Input: part model. Units: mm. Frame: model coordinates. A direction names the side the tool comes from. Coordinates: 2 decimals unless noted, no trailing zeros. Write each loop counter-clockwise with the first axis right and the second up, starting at its lowest first coordinate (ties: lowest second). Pieces come first, ordered by that corner, then holes. Notation, with made-up numbers: (48, 0) - (56, 0) arc R34 ccw to (56, 36) - close; hole circle Ø9 at (20.25, 25.25). An arc over 180 degrees is marked (long way). Use a Markdown table: item, result. Add a question column.
Q1. Pin query (flat end, axial travel): P1, Ø1.5, axis at y = 1.5, z = -10, coming from the +X side; P2, Ø0.7, axis at y = 8, z = 34.5, coming from the +X side; P3, Ø1.6, axis at x = 51, y = 0.5, coming from the -Z side. Return the tip coordinate at first contact, or that it passes through.
Q2. Section query B-B (x = 12). Return the cut outline in (y, z).
Q3. Mould query, pull axis Z, two halves, no side actions, for faces 4 (the face through (-14, 17.76, 34)), 5 (the face through (60.116, 10.483, 34.289)), 6 (the face through (-36, 1, -11)), 7 (the face through (35, 3.36, 23)). Classes: released by +Z, released by -Z, zero draft, split by the parting line, or undercut.
Q4. Set-up query: faces 1 (the face through (-39, 1, -5.32)), 2 (the face through (-52, 5.76, 23)), 3 (the face through (-57.11, 1.66, -19.82)). Return all of +Z, -Z, +X, -X, +Y, -Y with unobstructed straight access to the full face (end or side cutting, diameter ignored); none if empty.
Q5. Section query A-A (z = 6). Return the cut outline in (x, y).
Q6. Material intervals for probe 1 along Z at (x, y) = (-6.5, 11.75); probe 2 along Z at (x, y) = (30, 6.5); probe 3 along X at (y, z) = (16.75, 16), sorted ascending. Write a range as from..to.
Q7. Section query C-C (x = -40). Return the cut outline in (y, z).
Q8. Section query D-D (x = -24). Return the cut outline in (y, z).
from build123d import *

# Parameters (mm, degrees)
SKETCH_1_W           = 123.84
SKETCH_1_H           = 72
EXTRUDE_1_DEPTH      = 17.76
SKETCH_8_W           = 119.04
SKETCH_8_H           = 67.2
CUT_EXTRUDE_5_DEPTH  = 15.36
SKETCH_10_W          = 54.72
SKETCH_10_H          = 33.6
EXTRUDE_2_DEPTH      = 9.64
SKETCH_11_W          = 15
SKETCH_11_H          = 10.56
CUT_EXTRUDE_7_DEPTH  = 5
SKETCH_12_W          = 51.36
SKETCH_12_H          = 30.24
CUT_EXTRUDE_8_DEPTH  = 7
SKETCH_13_W          = 24.6
SKETCH_13_H          = 20.96
CUT_EXTRUDE_9_DEPTH  = 2
CUT_EXTRUDE_16_DEPTH = 73.428336996
FILLET_1_R           = 6
FILLET_3_R           = 3
FILLET_5_R           = 6
SKETCH_19_W          = 5.5
SKETCH_19_H          = 2
CUT_EXTRUDE_14_DEPTH = 3.84
SKETCH_20_W          = 5.5
SKETCH_20_H          = 2
CUT_EXTRUDE_15_DEPTH = 3.84
EXTRUDE_3_DEPTH      = 3.36
EXTRUDE_4_DEPTH      = 3.36
SKETCH_25_R          = 2.16
SKETCH_25_R_2        = 2.26
CUT_EXTRUDE_17_DEPTH = 74.793658264
SKETCH_22_R          = 3.71
SKETCH_22_R_2        = 3.12
CUT_EXTRUDE_18_DEPTH = 3.36
SKETCH_26_W          = 24.96
SKETCH_26_H          = 11.04
SKETCH_26_W_2        = 3.84
SKETCH_26_H_2        = 1.92
SKETCH_26_W_3        = 8.16
SKETCH_26_H_3        = 8.16
CUT_EXTRUDE_19_DEPTH = 74.793658264


with BuildPart() as part:
    # Эскиз1 → Бобышка-Вытянуть1 (new body)
    with BuildSketch(Plane(origin=(0, 0, 0), x_dir=(1, 0, 0), z_dir=(0, 1, 0))):
        Rectangle(SKETCH_1_W, SKETCH_1_H)
    extrude(amount=EXTRUDE_1_DEPTH)

    # Эскиз8 → Вырез-Вытянуть5 (cut)
    with BuildSketch(Plane(origin=(0, 17.76, 0), x_dir=(1, 0, 0), z_dir=(0, 1, 0))):
        Rectangle(SKETCH_8_W, SKETCH_8_H)
    extrude(amount=-CUT_EXTRUDE_5_DEPTH, mode=Mode.SUBTRACT)

    # Эскиз10 → Бобышка-Вытянуть2 (add)
    with BuildSketch(Plane(origin=(0, 2.4, 0), x_dir=(1, 0, 0), z_dir=(0, 1, 0))):
        with Locations((14.88, -2.2)):
            Rectangle(SKETCH_10_W, SKETCH_10_H)
    extrude(amount=EXTRUDE_2_DEPTH)

    # Эскиз11 → Вырез-Вытянуть7 (cut)
    with BuildSketch(Plane.XY.offset(33.6)):
        with Locations((-42.42, 9.12)):
            Rectangle(SKETCH_11_W, SKETCH_11_H)
    extrude(amount=CUT_EXTRUDE_7_DEPTH, mode=Mode.SUBTRACT)

    # Эскиз12 → Вырез-Вытянуть8 (cut)
    with BuildSketch(Plane.XZ):
        with Locations((14.64, 2.44)):
            Rectangle(SKETCH_12_W, SKETCH_12_H)
    extrude(amount=-CUT_EXTRUDE_8_DEPTH, mode=Mode.SUBTRACT)

    # Эскиз13 → Вырез-Вытянуть9 (cut)
    with BuildSketch(Plane.XZ):
        with Locations((49.62, 2.28)):
            Rectangle(SKETCH_13_W, SKETCH_13_H)
    extrude(amount=-CUT_EXTRUDE_9_DEPTH, mode=Mode.SUBTRACT)

    # Эскиз21 → Вырез-Вытянуть16 (cut, through all)
    with BuildSketch(Plane.XZ.offset(-7)):
        Polygon((-1.44, 7.24), (-1.44, -2.04), (-11.04, -2.04), (-11.04, 2.44), (-11.04, 7.24), align=None)
    extrude(amount=-CUT_EXTRUDE_16_DEPTH, mode=Mode.SUBTRACT)

    # Скругление1
    fillet_1_edges = [part.edges().sort_by_distance(p)[0] for p in [
        (-61.92, 8.88, -36),
        (61.92, 8.88, -36),
        (61.92, 8.88, 36),
        (-61.92, 8.88, 36),
    ]]
    fillet(fillet_1_edges, radius=FILLET_1_R)

    # Скругление3
    # the kernel refuses this fillet: 3 mm, written as the material it takes off along each edge
    with BuildSketch(Plane(origin=(55.92, 0, -30), x_dir=(1, 0, 0), z_dir=(0, 0, 1))) as fillet_3_piece_1:
        with BuildLine():
            CenterArc((6 - FILLET_3_R, FILLET_3_R), FILLET_3_R, 270, 90)
            Line((6, FILLET_3_R), (6 + FILLET_3_R * 0.02, FILLET_3_R))
            Line((6 + FILLET_3_R * 0.02, FILLET_3_R), (6 + FILLET_3_R * 0.02, -FILLET_3_R * 0.02))
            Line((6 + FILLET_3_R * 0.02, -FILLET_3_R * 0.02), (6 - FILLET_3_R, -FILLET_3_R * 0.02))
            Line((6 - FILLET_3_R, -FILLET_3_R * 0.02), (6 - FILLET_3_R, 0))
        make_face()
    revolve(axis=Axis((55.92, 0, -30), (0, 1, 0)), revolution_arc=90, mode=Mode.SUBTRACT)
    with BuildSketch(Plane(origin=(-55.92, 0, -36), x_dir=(0, 0, 1), z_dir=(1, 0, 0))) as fillet_3_piece_2:
        with BuildLine():
            CenterArc((FILLET_3_R, -FILLET_3_R), FILLET_3_R, 90, 90)
            Line((0, -FILLET_3_R), (-FILLET_3_R * 0.02, -FILLET_3_R))
            Line((-FILLET_3_R * 0.02, -FILLET_3_R), (-FILLET_3_R * 0.02, FILLET_3_R * 0.02))
            Line((-FILLET_3_R * 0.02, FILLET_3_R * 0.02), (FILLET_3_R, FILLET_3_R * 0.02))
            Line((FILLET_3_R, FILLET_3_R * 0.02), (FILLET_3_R, 0))
        make_face()
    extrude(amount=111.84, mode=Mode.SUBTRACT)
    with BuildSketch(Plane(origin=(-55.92, 0, -30), x_dir=(-1, 0, 0), z_dir=(0, 0, 1))) as fillet_3_piece_3:
        with BuildLine():
            CenterArc((6 - FILLET_3_R, -FILLET_3_R), FILLET_3_R, 0, 90)
            Line((6, -FILLET_3_R), (6 + FILLET_3_R * 0.02, -FILLET_3_R))
            Line((6 + FILLET_3_R * 0.02, -FILLET_3_R), (6 + FILLET_3_R * 0.02, FILLET_3_R * 0.02))
            Line((6 + FILLET_3_R * 0.02, FILLET_3_R * 0.02), (6 - FILLET_3_R, FILLET_3_R * 0.02))
            Line((6 - FILLET_3_R, FILLET_3_R * 0.02), (6 - FILLET_3_R, 0))
        make_face()
    revolve(axis=Axis((-55.92, 0, -30), (0, -1, 0)), revolution_arc=90, mode=Mode.SUBTRACT)
    with BuildSketch(Plane(origin=(-61.92, 0, 30), x_dir=(1, 0, 0), z_dir=(0, 0, -1))) as fillet_3_piece_4:
        with BuildLine():
            CenterArc((FILLET_3_R, -FILLET_3_R), FILLET_3_R, 90, 90)
            Line((0, -FILLET_3_R), (-FILLET_3_R * 0.02, -FILLET_3_R))
            Line((-FILLET_3_R * 0.02, -FILLET_3_R), (-FILLET_3_R * 0.02, FILLET_3_R * 0.02))
            Line((-FILLET_3_R * 0.02, FILLET_3_R * 0.02), (FILLET_3_R, FILLET_3_R * 0.02))
            Line((FILLET_3_R, FILLET_3_R * 0.02), (FILLET_3_R, 0))
        make_face()
    extrude(amount=60, mode=Mode.SUBTRACT)
    with BuildSketch(Plane(origin=(-55.92, 0, 30), x_dir=(0, 0, 1), z_dir=(1, 0, 0))) as fillet_3_piece_5:
        with BuildLine():
            CenterArc((6 - FILLET_3_R, -FILLET_3_R), FILLET_3_R, 0, 90)
            Line((6, -FILLET_3_R), (6 + FILLET_3_R * 0.02, -FILLET_3_R))
            Line((6 + FILLET_3_R * 0.02, -FILLET_3_R), (6 + FILLET_3_R * 0.02, FILLET_3_R * 0.02))
            Line((6 + FILLET_3_R * 0.02, FILLET_3_R * 0.02), (6 - FILLET_3_R, FILLET_3_R * 0.02))
            Line((6 - FILLET_3_R, FILLET_3_R * 0.02), (6 - FILLET_3_R, 0))
        make_face()
    revolve(axis=Axis((-55.92, 0, 30), (0, -1, 0)), revolution_arc=90, mode=Mode.SUBTRACT)
    with BuildSketch(Plane(origin=(61.92, 0, -5.24), x_dir=(-1, 0, 0), z_dir=(0, 0, 1))) as fillet_3_piece_6:
        with BuildLine():
            CenterArc((FILLET_3_R, -FILLET_3_R), FILLET_3_R, 90, 90)
            Line((0, -FILLET_3_R), (-FILLET_3_R * 0.02, -FILLET_3_R))
            Line((-FILLET_3_R * 0.02, -FILLET_3_R), (-FILLET_3_R * 0.02, FILLET_3_R * 0.02))
            Line((-FILLET_3_R * 0.02, FILLET_3_R * 0.02), (FILLET_3_R, FILLET_3_R * 0.02))
            Line((FILLET_3_R, FILLET_3_R * 0.02), (FILLET_3_R, 0))
        make_face()
    extrude(amount=35.24, mode=Mode.SUBTRACT)
    with BuildSketch(Plane(origin=(55.92, 0, 30), x_dir=(0, 0, 1), z_dir=(-1, 0, 0))) as fillet_3_piece_7:
        with BuildLine():
            CenterArc((6 - FILLET_3_R, FILLET_3_R), FILLET_3_R, 270, 90)
            Line((6, FILLET_3_R), (6 + FILLET_3_R * 0.02, FILLET_3_R))
            Line((6 + FILLET_3_R * 0.02, FILLET_3_R), (6 + FILLET_3_R * 0.02, -FILLET_3_R * 0.02))
            Line((6 + FILLET_3_R * 0.02, -FILLET_3_R * 0.02), (6 - FILLET_3_R, -FILLET_3_R * 0.02))
            Line((6 - FILLET_3_R, -FILLET_3_R * 0.02), (6 - FILLET_3_R, 0))
        make_face()
    revolve(axis=Axis((55.92, 0, 30), (0, 1, 0)), revolution_arc=90, mode=Mode.SUBTRACT)
    with BuildSketch(Plane(origin=(55.92, 0, 36), x_dir=(0, 1, 0), z_dir=(-1, 0, 0))) as fillet_3_piece_8:
        with BuildLine():
            CenterArc((FILLET_3_R, FILLET_3_R), FILLET_3_R, 180, 90)
            Line((0, FILLET_3_R), (-FILLET_3_R * 0.02, FILLET_3_R))
            Line((-FILLET_3_R * 0.02, FILLET_3_R), (-FILLET_3_R * 0.02, -FILLET_3_R * 0.02))
            Line((-FILLET_3_R * 0.02, -FILLET_3_R * 0.02), (FILLET_3_R, -FILLET_3_R * 0.02))
            Line((FILLET_3_R, -FILLET_3_R * 0.02), (FILLET_3_R, 0))
        make_face()
    extrude(amount=111.84, mode=Mode.SUBTRACT)
    with BuildSketch(Plane(origin=(61.92, 0, -30), x_dir=(-1, 0, 0), z_dir=(0, 0, 1))) as fillet_3_piece_9:
        with BuildLine():
            CenterArc((FILLET_3_R, -FILLET_3_R), FILLET_3_R, 90, 90)
            Line((0, -FILLET_3_R), (-FILLET_3_R * 0.02, -FILLET_3_R))
            Line((-FILLET_3_R * 0.02, -FILLET_3_R), (-FILLET_3_R * 0.02, FILLET_3_R * 0.02))
            Line((-FILLET_3_R * 0.02, FILLET_3_R * 0.02), (FILLET_3_R, FILLET_3_R * 0.02))
            Line((FILLET_3_R, FILLET_3_R * 0.02), (FILLET_3_R, 0))
        make_face()
    extrude(amount=39.8, mode=Mode.SUBTRACT)

    # Скругление5
    fillet_5_edges = [part.edges().sort_by_distance(p)[0] for p in [
        (-59.52, 10.08, 33.6),
        (-59.52, 10.08, -33.6),
        (59.52, 10.08, -33.6),
        (59.52, 10.08, 33.6),
    ]]
    fillet(fillet_5_edges, radius=FILLET_5_R)

    # Эскиз19 → Вырез-Вытянуть14 (cut)
    with BuildSketch(Plane(origin=(0, 0, 17.56), x_dir=(-1, 0, 0), z_dir=(0, 0, -1))):
        with Locations((2.75, 3)):
            Rectangle(SKETCH_19_W, SKETCH_19_H)
    extrude(amount=-CUT_EXTRUDE_14_DEPTH, mode=Mode.SUBTRACT)

    # Эскиз20 → Вырез-Вытянуть15 (cut)
    with BuildSketch(Plane.XY.offset(-12.68)):
        with Locations((-2.75, 3)):
            Rectangle(SKETCH_20_W, SKETCH_20_H)
    extrude(amount=-CUT_EXTRUDE_15_DEPTH, mode=Mode.SUBTRACT)

    # Эскиз24 → Бобышка-Вытянуть3 (add)
    with BuildSketch(Plane(origin=(0, 2.4, 0), x_dir=(1, 0, 0), z_dir=(0, 1, 0))):
        with BuildLine():
            Line((32.198823657, -19), (43.081176343, -19))
            ThreePointArc((43.081176343, -19), (37.64, -29.28), (32.198823657, -19))
        make_face()
        with BuildLine():
            Line((32.198823657, 14.6), (43.075947447, 14.592322107))
            ThreePointArc((43.075947447, 14.592322107), (37.644644658, 24.879998361), (32.198823657, 14.6))
        make_face()
    extrude(amount=EXTRUDE_3_DEPTH)

    # Эскиз23 → Бобышка-Вытянуть4 (add)
    with BuildSketch(Plane(origin=(0, 2.4, 0), x_dir=(1, 0, 0), z_dir=(0, 1, 0))):
        with BuildLine():
            Line((-59.52, 25.73022458), (-59.52, 17.26977542))
            ThreePointArc((-59.52, 17.26977542), (-47.9, 21.5), (-59.52, 25.73022458))
        make_face()
        with BuildLine():
            Line((-59.52, -25.73022458), (-59.52, -17.26977542))
            ThreePointArc((-59.52, -17.26977542), (-47.9, -21.5), (-59.52, -25.73022458))
        make_face()
    extrude(amount=EXTRUDE_4_DEPTH)

    # Эскиз25 → Вырез-Вытянуть17 (cut, through all)
    with BuildSketch(Plane(origin=(0, 0, 0), x_dir=(1, 0, 0), z_dir=(0, 1, 0))):
        with Locations(Location((-54.48, -21.5, 0), (0, 0, 270))):
            Circle(SKETCH_25_R)
        with Locations(Location((-54.48, 21.5, 0), (0, 0, 270))):
            Circle(SKETCH_25_R)
        with Locations(Location((37.64, 18.3, 0), (0, 0, 90))):
            Circle(SKETCH_25_R_2)
        with Locations(Location((37.64, -22.7, 0), (0, 0, 90))):
            Circle(SKETCH_25_R_2)
    extrude(amount=CUT_EXTRUDE_17_DEPTH, mode=Mode.SUBTRACT)

    # Эскиз22 → Вырез-Вытянуть18 (cut)
    with BuildSketch(Plane.XZ):
        with Locations(Location((37.64, -18.3, 0), (0, 0, 270))):
            Circle(SKETCH_22_R)
        with Locations(Location((37.64, 22.7, 0), (0, 0, 270))):
            Circle(SKETCH_22_R)
        with Locations(Location((-54.48, 21.5, 0), (0, 0, 90))):
            Circle(SKETCH_22_R_2)
        with Locations(Location((-54.48, -21.5, 0), (0, 0, 90))):
            Circle(SKETCH_22_R_2)
    extrude(amount=-CUT_EXTRUDE_18_DEPTH, mode=Mode.SUBTRACT)

    # Эскиз26 → Вырез-Вытянуть19 (cut, through all)
    with BuildSketch(Plane.XZ):
        with Locations((12.761591223, -23.48)):
            Rectangle(SKETCH_26_W, SKETCH_26_H)
        with Locations((-35.56, -10.04)):
            Rectangle(SKETCH_26_W_2, SKETCH_26_H_2)
        with Locations((-38.96, -1.24)):
            Rectangle(SKETCH_26_W_3, SKETCH_26_H_3)
    extrude(amount=-CUT_EXTRUDE_19_DEPTH, mode=Mode.SUBTRACT)


solid = part.part
Values follow:
| question | item | result |
|---|---|---|
| 1 | P1 | x = 61.82 |
| 1 | P2 | x = 60.25 |
| 1 | P3 | z = -35.47 |
| 2 | outline | (0, -33) arc R3 ccw to (3, -36) - (17.76, -36) - (17.76, -33.6) - (2.4, -33.6) - (2.4, -29) - (0, -29) - close; (0, -17.96) - (2.4, -17.96) - (2.4, -14.6) - (12.04, -14.6) - (12.04, 19) - (2.4, 19) - (2.4, 33.6) - (17.76, 33.6) - (17.76, 36) - (3, 36) arc R3 ccw to (0, 33) - (0, 17.56) - (7, 17.56) - (7, -12.68) - (0, -12.68) - close |
| 3 | face 4 | zero draft |
| 3 | face 5 | released by +Z |
| 3 | face 6 | undercut |
| 3 | face 7 | undercut |
| 4 | face 1 | +Y, -Y |
| 4 | face 2 | +Y |
| 4 | face 3 | -Y |
| 5 | outline | (-61.92, 3) arc R3 ccw to (-58.92, 0) - (-11.04, 0) - (-11.04, 12.04) - (-12.48, 12.04) - (-12.48, 2.4) - (-59.52, 2.4) - (-59.52, 17.76) - (-61.92, 17.76) - close; (-1.44, 7) - (40.32, 7) - (40.32, 2) - (61.75, 2) arc R3 ccw to (61.92, 3) - (61.92, 17.76) - (59.52, 17.76) - (59.52, 2.4) - (42.24, 2.4) - (42.24, 12.04) - (-1.44, 12.04) - close |
| 6 | probe 1 | -36..-33.6, -14.6..-2.04, 7.24..19, 33.6..36 |
| 6 | probe 2 | -36..-33.6, -14.6..-12.68, 17.56..19, 33.6..36 |
| 6 | probe 3 | -61.92..-59.52, 59.52..61.92 |
| 7 | outline | (0, -33) arc R3 ccw to (3, -36) - (17.76, -36) - (17.76, -33.6) - (2.4, -33.6) - (2.4, -5.32) - (0, -5.32) - close; (0, 2.84) - (2.4, 2.84) - (2.4, 33.6) - (3.84, 33.6) - (3.84, 36) - (3, 36) arc R3 ccw to (0, 33) - close; (14.4, 33.6) - (17.76, 33.6) - (17.76, 36) - (14.4, 36) - close |
| 8 | outline | (0, -33) arc R3 ccw to (3, -36) - (17.76, -36) - (17.76, -33.6) - (2.4, -33.6) - (2.4, 33.6) - (17.76, 33.6) - (17.76, 36) - (3, 36) arc R3 ccw to (0, 33) - close |
